```python
from build123d import *

# Parameters (mm, degrees)
SKETCH1_W           = 75
SKETCH1_H           = 65
BOSS_EXTRUDE1_DEPTH = 22
SKETCH2_W           = 55
SKETCH2_H           = 12
CUT_EXTRUDE1_DEPTH  = 70
SKETCH3_W           = 15
SKETCH3_H           = 12
CUT_EXTRUDE2_DEPTH  = 85.647799735
SKETCH4_R           = 1.75
CUT_EXTRUDE3_DEPTH  = 55.281672782
SKETCH7_R           = 1.75
CUT_EXTRUDE5_DEPTH  = 55.281672782
SKETCH8_R           = 1.75
CUT_EXTRUDE6_DEPTH  = 55.281672782
SKETCH9_R           = 3.5
CUT_EXTRUDE7_DEPTH  = 6
SKETCH10_R          = 3.5
CUT_EXTRUDE8_DEPTH  = 6


with BuildPart() as part:
    # Sketch1 → Boss-Extrude1 (new body)
    with BuildSketch(Plane(origin=(0, 0, 0), x_dir=(1, 0, 0), z_dir=(0, 1, 0))):
        Rectangle(SKETCH1_W, SKETCH1_H)
    extrude(amount=BOSS_EXTRUDE1_DEPTH)

    # Sketch2 → Cut-Extrude1 (cut)
    with BuildSketch(Plane(origin=(37.5, 0, 0), x_dir=(0, 0, -1), z_dir=(1, 0, 0))):
        with Locations((0, 11)):
            Rectangle(SKETCH2_W, SKETCH2_H)
    extrude(amount=-CUT_EXTRUDE1_DEPTH, mode=Mode.SUBTRACT)

    # Sketch3 → Cut-Extrude2 (cut, through all)
    with BuildSketch(Plane.ZY.offset(37.5)):
        with Locations((-17, 11)):
            Rectangle(SKETCH3_W, SKETCH3_H)
    extrude(amount=-CUT_EXTRUDE2_DEPTH, mode=Mode.SUBTRACT)

    # Sketch4 → Cut-Extrude3 (cut, through all)
    with BuildSketch(Plane(origin=(0, 22, 0), x_dir=(1, 0, 0), z_dir=(0, 1, 0))):
        with Locations(Location((19, -25, 0), (0, 0, 270))):
            Circle(SKETCH4_R)
    extrude(amount=-CUT_EXTRUDE3_DEPTH, mode=Mode.SUBTRACT)

    # Sketch7 → Cut-Extrude5 (cut, through all)
    with BuildSketch(Plane(origin=(0, 22, 0), x_dir=(1, 0, 0), z_dir=(0, 1, 0))):
        with Locations(Location((19, 23.5, 0), (0, 0, 270))):
            Circle(SKETCH7_R)
    extrude(amount=-CUT_EXTRUDE5_DEPTH, mode=Mode.SUBTRACT)

    # Sketch8 → Cut-Extrude6 (cut, through all)
    with BuildSketch(Plane(origin=(0, 22, 0), x_dir=(1, 0, 0), z_dir=(0, 1, 0))):
        with Locations(Location((-29.5, -10, 0), (0, 0, 270))):
            Circle(SKETCH8_R)
    extrude(amount=-CUT_EXTRUDE6_DEPTH, mode=Mode.SUBTRACT)

    # Sketch9 → Cut-Extrude7 (cut)
    with BuildSketch(Plane(origin=(0, 22, 0), x_dir=(1, 0, 0), z_dir=(0, 1, 0))):
        with Locations(Location((0, -16.25, 0), (0, 0, 270))):
            Circle(SKETCH9_R)
    extrude(amount=-CUT_EXTRUDE7_DEPTH, mode=Mode.SUBTRACT)

    # Sketch10 → Cut-Extrude8 (cut)
    with BuildSketch(Plane(origin=(0, 22, 0), x_dir=(1, 0, 0), z_dir=(0, 1, 0))):
        with Locations(Location((0, 16.25, 0), (0, 0, 270))):
            Circle(SKETCH10_R)
    extrude(amount=-CUT_EXTRUDE8_DEPTH, mode=Mode.SUBTRACT)


solid = part.part
```
Read the model definition and answer for the solid it produces. Units are mm, in the model's axes. A direction names the side the tool comes from. Round coordinates to 2 decimals unless told otherwise and drop trailing zeros. Write each loop counter-clockwise with the first axis right and the second up, starting at its lowest first coordinate (ties: lowest second). Pieces come first, ordered by that corner, then holes. Notation, with made-up numbers: (49, 48) -> (99, 48) arc R12 cw to (99, 70) -> close; hole circle Ø4 at (-32.75, 62.25). An arc over 180 degrees is marked (long way). Answer in a Markdown table with one row per item. Add a question column.
1) Consider line 1 (X direction, y = 18.6, z = -23.5); line 2 (Y direction, x = -11, z = -6); line 3 (Z direction, x = 31, y = 10). Determine where each line is inside the solid, lowest interval first.
2) Find section C-C, the plane y = 7.5. Determine the outline of the cut face in (x, z).
3) Find section D-D, the plane x = 0. Determine the outline of the cut face in (y, z).
4) Which of the six approach directions +Z, -Z, +X, -X, +Y, -Y give full straight-line access (tool end or side, diameter ignored) to faces 4 (the face through (-35, 11, -9.5)), 5 (the face through (3, 11, 27.5)), 6 (the face through (1.05, 19.54, 19.59)), 7 (the face through (-37.5, 11, 0))?
5) Find section A-A, the plane z = 16.25. Determine the outline of the cut face in (x, y), and give its area (3 significant figures).
6) Find section B-B, the plane x = 19. Determine the outline of the cut face in (y, z), and give its area (3 significant figures).
7) Determine the mould class of faces 1 (the face through (-1, 11, 32.5)), 2 (the face through (20.18, 2.54, -24.79)), 3 (the face through (-1, 0, 0)) for opening direction Z: pulls with the +Z half, pulls with the -Z half, needs draft (parallel to the pull), parting line crosses it, or undercut.
8) Given P1, Ø2.5, axis at y = 12, z = -26, coming from the +X side, flat-ended and moving along its own axis, determine where the tip first touches the part or whether it passes through.
Findings below:
| question | item | result |
|---|---|---|
| 1 | line 1 | -37.5 to 17.25, 20.75 to 37.5 |
| 1 | line 2 | 0 to 5, 17 to 22 |
| 1 | line 3 | -32.5 to -27.5, 27.5 to 32.5 |
| 2 | outline | (-37.5, -32.5) -> (37.5, -32.5) -> (37.5, -27.5) -> (-32.5, -27.5) -> (-32.5, -24.5) -> (-37.5, -24.5) -> close; (-37.5, -9.5) -> (-32.5, -9.5) -> (-32.5, 27.5) -> (37.5, 27.5) -> (37.5, 32.5) -> (-37.5, 32.5) -> close |
| 3 | outline | (0, -32.5) -> (22, -32.5) -> (22, -19.75) -> (17, -19.75) -> (17, -27.5) -> (5, -27.5) -> (5, 27.5) -> (17, 27.5) -> (17, 19.75) -> (22, 19.75) -> (22, 32.5) -> (0, 32.5) -> close; (17, -12.75) -> (22, -12.75) -> (22, 12.75) -> (17, 12.75) -> close |
| 4 | face 4 | +X, -X |
| 4 | face 5 | +X |
| 4 | face 6 | +Y |
| 4 | face 7 | +Z, -Z, -X, +Y, -Y |
| 5 | outline | (-37.5, 0) -> (37.5, 0) -> (37.5, 5) -> (-32.5, 5) -> (-32.5, 17) -> (-3.5, 17) -> (-3.5, 22) -> (-37.5, 22) -> close; (3.5, 17) -> (37.5, 17) -> (37.5, 22) -> (3.5, 22) -> close |
| 5 | area | 775 mm² |
| 6 | outline | (0, -32.5) -> (22, -32.5) -> (22, -25.25) -> (17, -25.25) -> (17, -27.5) -> (5, -27.5) -> (5, -25.25) -> (0, -25.25) -> close; (0, -21.75) -> (5, -21.75) -> (5, 23.25) -> (0, 23.25) -> close; (0, 26.75) -> (5, 26.75) -> (5, 27.5) -> (17, 27.5) -> (17, 26.75) -> (22, 26.75) -> (22, 32.5) -> (0, 32.5) -> close; (17, -21.75) -> (22, -21.75) -> (22, 23.25) -> (17, 23.25) -> close |
| 6 | area | 700 mm² |
| 7 | face 1 | pulls with the +Z half |
| 7 | face 2 | undercut |
| 7 | face 3 | needs draft |
| 8 | P1 | x = -32.5 |
